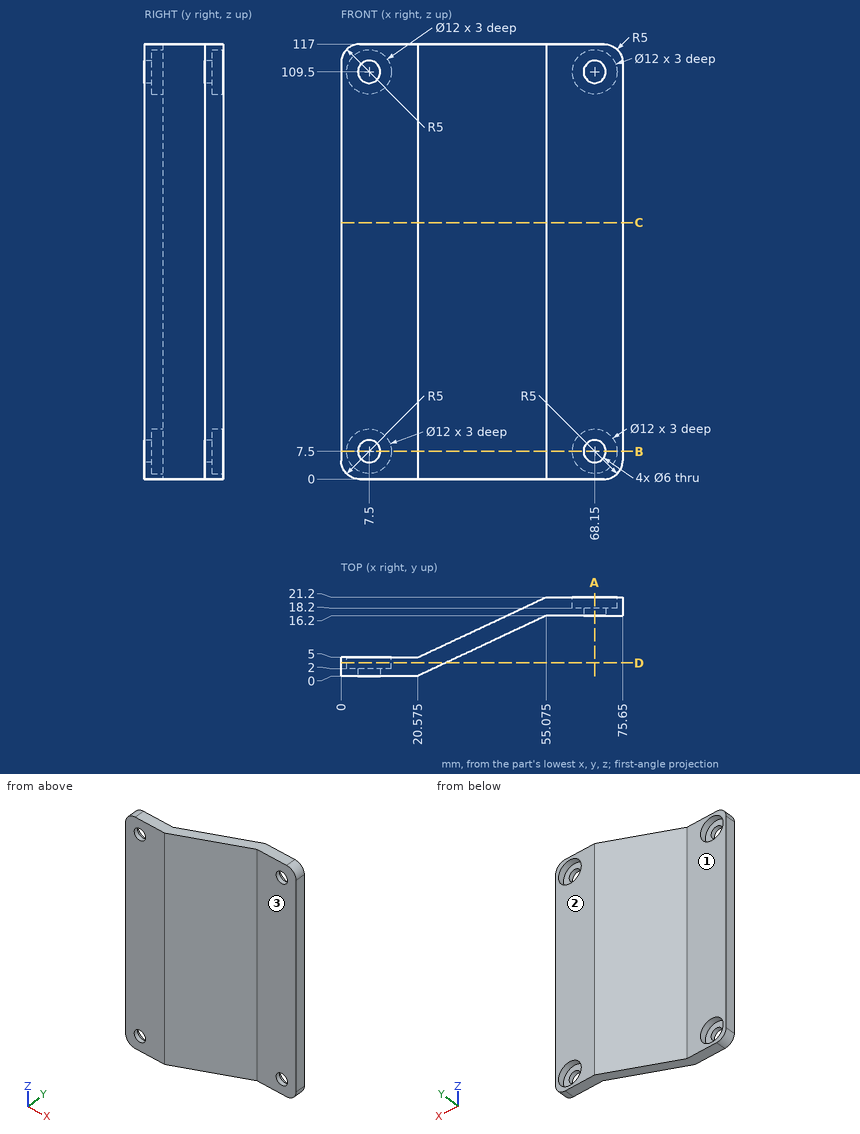
Study the drawing (mm; zero at the part's minimum x, y, z) and answer. A direction names the side the tool comes from. Coordinates: 2 decimals unless noted, no trailing zeros. Write each loop counter-clockwise with the first axis right and the second up, starting at its lowest first coordinate (ties: lowest second). Pieces come first, ordered by that corner, then holes.
Q1. A cutting plane is placed at B-B, the plane z = 7.5. Give the vertices of the cut face in (x, y) (3 decimals).
Q2. A cutting plane is placed at C-C, the plane z = 69. Give the vertices of the cut face in (x, y) (3 decimals).
Q3. Each of these flat-tipped pins is pushed along its axis until it touches: pin 1 Ø11 at (x, z) = (68.15, 7.5) entering from +Y; pin 2 Ø7 at (x, z) = (7.5, 109.5) entering from -Y; pin 3 Ø3.5 at (x, z) = (9, 10) entering from +Y; pin 4 Ø8 at (y, z) = (11.5, 72) entering from +X. Where does it stop, or does it pass through?
Q4. A cutting plane is placed at D-D, the plane y = 3.5. Give the vertices of the cut face in (x, z), then the cut area to 3 significant figures.
Q5. A cutting plane is placed at A-A, the plane x = 68.15. Give the vertices of the cut face in (y, z).
Q6. Which of the six approach directions +Z, -Z, +X, -X, +Y, -Y give full straight-line access (tool end or side, diameter ignored) to the marked faces 1, 2 and 3?
Q7. Find the intervals of material crossed by line 1 (Z direction, x = 7.5, y = 0.6); line 2 (Z direction, x = 68.15, y = 19.55); line 3 (Y direction, x = 58, z = 65), in increasing order.
Findings below:
1. outline: (0, 0) - (4.5, 0) - (4.5, 2) - (1.5, 2) - (1.5, 5) - (0, 5) - close; (10.5, 0) - (20.575, 0) - (55.075, 16.2) - (65.15, 16.2) - (65.15, 18.2) - (62.15, 18.2) - (62.15, 21.2) - (55.075, 21.2) - (20.575, 5) - (13.5, 5) - (13.5, 2) - (10.5, 2) - close; (71.15, 16.2) - (75.65, 16.2) - (75.65, 21.2) - (74.15, 21.2) - (74.15, 18.2) - (71.15, 18.2) - close
2. outline: (0, 0) - (20.575, 0) - (55.075, 16.2) - (75.65, 16.2) - (75.65, 21.2) - (55.075, 21.2) - (20.575, 5) - (0, 5) - close
3. pin 1: stops at y = 18.2
3. pin 2: stops at y = 0
3. pin 3: stops at y = 2
3. pin 4: stops at x = 53.58
4. outline: (0, 5) arc R5 ccw to (5, 0) - (28.03, 0) - (28.03, 117) - (5, 117) arc R5 ccw to (0, 112) - close; hole circle Ø12 at (7.5, 7.5); hole circle Ø12 at (7.5, 109.5)
4. area: 3,040 mm2
5. outline: (16.2, 0) - (21.2, 0) - (21.2, 1.5) - (18.2, 1.5) - (18.2, 4.5) - (16.2, 4.5) - close; (16.2, 10.5) - (18.2, 10.5) - (18.2, 13.5) - (21.2, 13.5) - (21.2, 103.5) - (18.2, 103.5) - (18.2, 106.5) - (16.2, 106.5) - close; (16.2, 112.5) - (18.2, 112.5) - (18.2, 115.5) - (21.2, 115.5) - (21.2, 117) - (16.2, 117) - close
6. face 1: +Z, -Z, -X, +Y
6. face 2: +Z, -Z, +X, -X, +Y
6. face 3: +Z, -Z, +X, -Y
7. line 1: z = 0 to 4.5, 10.5 to 106.5, 112.5 to 117
7. line 2: z = 0 to 1.5, 13.5 to 103.5, 115.5 to 117
7. line 3: y = 16.2 to 21.2
